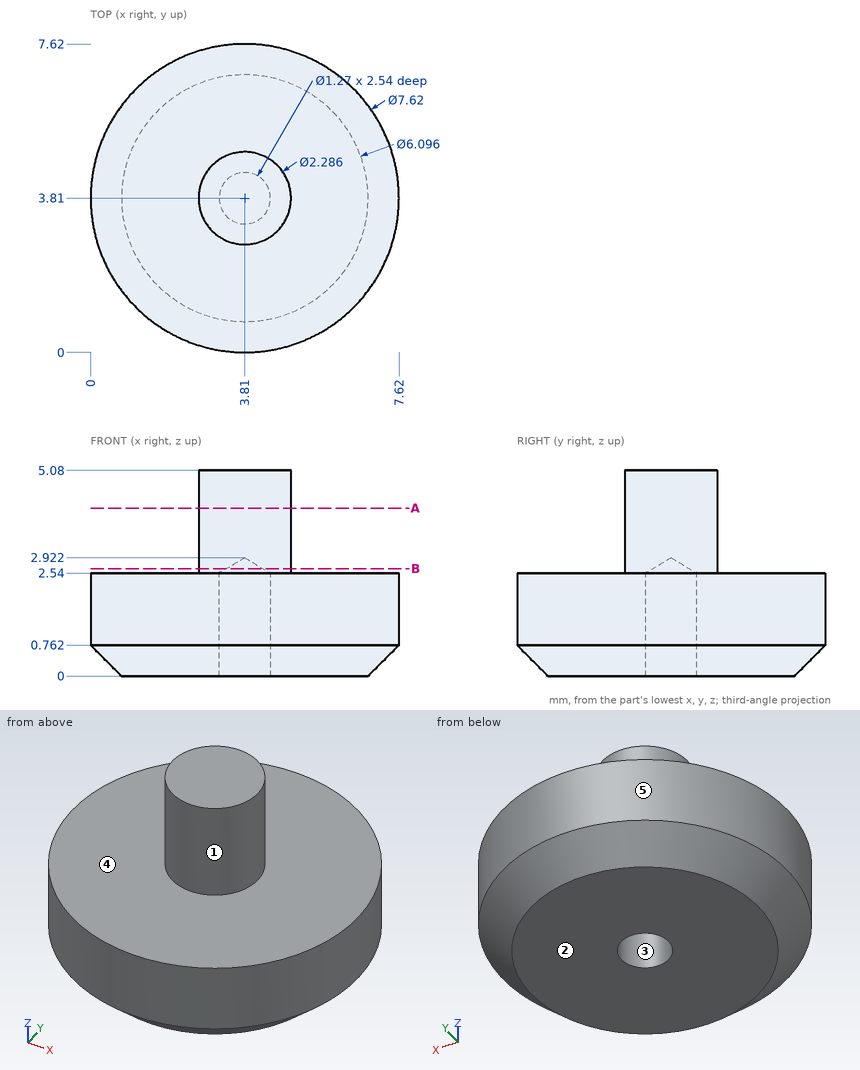
Can you work these out from the drawing? Everything is in mm from the part's minimum corner. A direction names the side the tool comes from. Coordinates: 2 decimals unless noted, no trailing zeros. Order: outer loops, then holes, each group sorted by start corner. A loop starts at its lowest first (then second) coordinate and runs counter-clockwise, first axis right, second up. Notation, with made-up numbers: M 80.25,47.25 L 108.25,47.25 A10 cw 108.25,62.25 Z; hole C 51,-28.5 d3. An arc over 180 degrees is marked long. Answer as CSV lines item,"result". Start each with the question number.
1. We'd pull the mould along X, two halves only. Please class the marked faces 3, 4 and 5: released by +X, released by -X, zero draft, split by the parting line, or undercut.
2. I want a section at B-B, the plane z = 2.65. Write out the boundary of the cut face in (x, y).
3. For pin 1 (3 mm diameter, centred on x = 6.5, y = 3.5, fed in from +Z), with a flat end and sliding along its axis, tell me the tip position at first contact or that it passes through.
4. I want a section at A-A, the plane z = 4.15. Write out the boundary of the cut face in (x, y).
5. I need wall thicknesses on line 1 (Y direction, x = 3.81, z = 1.6) (1 decimal); line 2 (Z direction, x = 5, y = 2.25); line 3 (X direction, y = 3.5, z = 2.5) (1 decimal). Which ranges of each line are inside material? Lowest first, please. Write a range as [from, to].
6. On a 3-axis mill with a long thin cutter (end or side, diameter ignored), from which of +Z, -Z, +X, -X, +Y, -Y can I reach the whole of each face in a straight line? I mean the marked faces 1 and 2. Say none if no direction works.
Recorded:
1,face 3,"undercut"
1,face 4,"zero draft"
1,face 5,"split by the parting line"
2,outline,"C 3.81,3.81 d2.29; hole C 3.81,3.81 d0.9"
3,pin 1,"stops at z = 2.54"
4,outline,"C 3.81,3.81 d2.29"
5,line 1,"y = [0, 3.2], [4.4, 7.6]"
5,line 2,"z = [0, 2.54]"
5,line 3,"x = [0, 3.3], [4.4, 7.6]"
6,face 1,"+Z"
6,face 2,"-Z, +X, -X, +Y, -Y"
